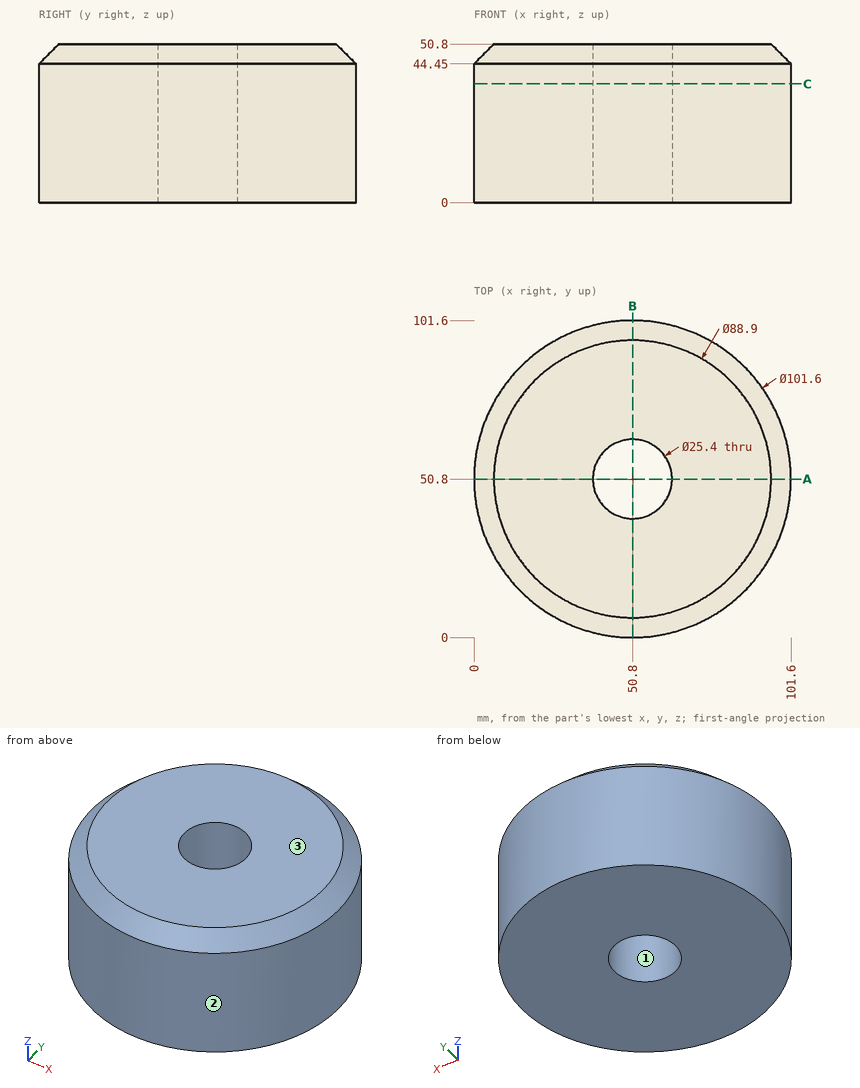
Geometry check sheet. Reference: drawing and pictorial views, mm from the part's lowest x, y, z. Round coordinates to 2 decimals unless told otherwise and drop trailing zeros. Order: outer loops, then holes, each group sorted by start corner. A loop starts at its lowest first (then second) coordinate and runs counter-clockwise, first axis right, second up. Notation, with made-up numbers: (8.5, 24) - (13.5, 24) arc R26 cw to (13.5, 45) - close; hole circle Ø2 at (-16, -16). An arc over 180 degrees is marked (long way). One line per question, with ' | ' between items. Start each with the question number.
(1) Release check for a two-part mould opening along Y. For the marked faces 1, 2 and 3 record: released by +Y, released by -Y, zero draft, split by the parting line, or undercut.
(2) Sectioned sample at A-A on y = 50.8. Record the cut outline in (x, z).
(3) Depth check by flat-ended pin: pin 1 Ø2 at (y, z) = (55.5, 34.5) entering from +X; pin 2 Ø6 at (y, z) = (18, 5) entering from +X; pin 3 Ø1.5 at (x, z) = (32, 16.5) entering from -Y; pin 4 Ø12 at (x, y) = (87, 85.5) entering from -Z. Enter the tip coordinate at first touch or a pass-through.
(4) Sectioned sample at C-C on z = 38. Record the cut outline in (x, y), and give its area (3 significant figures).
(5) Thickness scan on L1, parallel to Y at x = 50.8, z = 28; L2, parallel to Y at x = 40, z = 24; L3, parallel to Z at x = 89.5, y = 21. Record the ranges inside material, lowest first. Write a range as [from, to].
Conclusion:
1) face 1: undercut | face 2: split by the parting line | face 3: zero draft
2) outline: (0, 0) - (38.1, 0) - (38.1, 50.8) - (6.35, 50.8) - (0, 44.45) - close; (63.5, 0) - (101.6, 0) - (101.6, 44.45) - (95.25, 50.8) - (63.5, 50.8) - close
3) pin 1: stops at x = 101.47 | pin 2: stops at x = 91.94 | pin 3: stops at y = 3.31 | pin 4: stops at z = 0
4) outline: circle Ø101.6 at (50.8, 50.8); hole circle Ø25.4 at (50.8, 50.8) | area: 7,600 mm2
5) L1: y = [0, 38.1], [63.5, 101.6] | L2: y = [1.16, 44.12], [57.48, 100.44] | L3: z = [0, 46.41]
